Answer from the drawing. Dimensions are ordinates in mm from the lowest x, y and z of the part. Give positions to 0.01 mm unless a question says otherwise; leave off trailing zeros. Order: outer loops, then holes, each group sorted by start corner. A loop starts at its lowest first (then second) coordinate and runs counter-clockwise, first axis right, second up. Notation, with made-up numbers: (83.5, 46.25) - (142.5, 46.25) arc R17 ccw to (142.5, 62.25) - close; hole circle Ø11 at (-29, 48). An arc over 180 degrees is marked (long way). Answer in a Markdown table with one row per item.
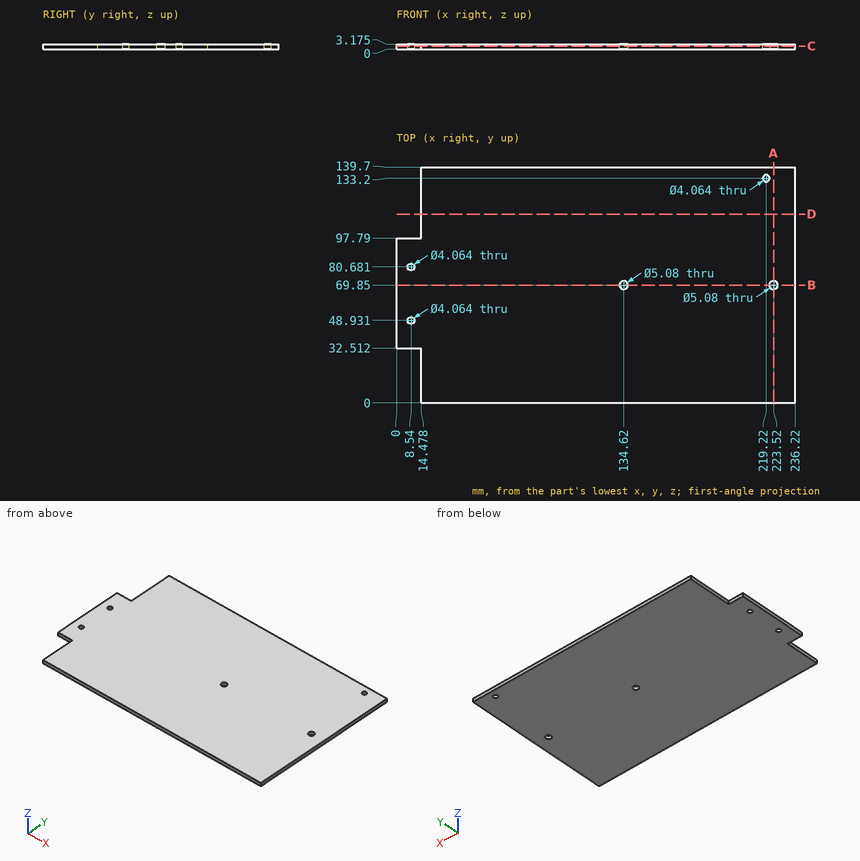
Item 1: Consider line 1 (Y direction, x = 134.62, z = 2.5); line 2 (X direction, y = 133.2, z = 2.05); line 3 (X direction, y = 68, z = 1.95). Determine where each line is inside the solid, lowest interval first.
Answer block:
| item | result |
|---|---|
| line 1 | 0 to 67.31, 72.39 to 139.7 |
| line 2 | 14.48 to 217.19, 221.25 to 236.22 |
| line 3 | 0 to 132.88, 136.36 to 221.78, 225.26 to 236.22 |
Item 2: Find section D-D on y = 112. Write down the section's boundary in (x, z) (1 decimal), then the cut area to 3 significant figures.
Answer block:
| item | result |
|---|---|
| outline | (14.5, 0) - (236.2, 0) - (236.2, 3.2) - (14.5, 3.2) - close |
| area | 704 mm² |
Item 3: This flat-tipped pin is pushed along its axis until it touches: P1, Ø1.6, axis at y = 109.5, z = 2, coming from the -X side. Where does it stop, or does it pass through?
Answer block:
| item | result |
|---|---|
| P1 | x = 14.48 |
Item 4: Find section A-A on x = 223.52. Write down the section's boundary in (y, z) (1 decimal).
Answer block:
| item | result |
|---|---|
| outline | (0, 0) - (67.3, 0) - (67.3, 3.2) - (0, 3.2) - close; (72.4, 0) - (139.7, 0) - (139.7, 3.2) - (72.4, 3.2) - close |
Item 5: Find section B-B on y = 69.85. Write down the section's boundary in (x, z) (1 decimal).
Answer block:
| item | result |
|---|---|
| outline | (0, 0) - (132.1, 0) - (132.1, 3.2) - (0, 3.2) - close; (137.2, 0) - (221, 0) - (221, 3.2) - (137.2, 3.2) - close; (226.1, 0) - (236.2, 0) - (236.2, 3.2) - (226.1, 3.2) - close |
Item 6: Find section C-C on z = 1.9. Write down the section's boundary in (x, y).
Answer block:
| item | result |
|---|---|
| outline | (0, 32.51) - (14.48, 32.51) - (14.48, 0) - (236.22, 0) - (236.22, 139.7) - (14.48, 139.7) - (14.48, 97.79) - (0, 97.79) - close; hole circle Ø4.06 at (8.54, 48.93); hole circle Ø4.06 at (8.54, 80.68); hole circle Ø5.08 at (134.62, 69.85); hole circle Ø4.06 at (219.22, 133.2); hole circle Ø5.08 at (223.52, 69.85) |
